from build123d import *

# Parameters (mm, degrees)
F0_W      = 139.7
F0_H      = 19.05
F1_DEPTH  = 6.35
F2_R      = 3.175
F3_DEPTH  = 6.351
F4_R      = 3.175
F5_DEPTH  = 25.4
F6_R      = 9.52499
F7_R      = 9.52499
F8_R      = 3.175
F9_DEPTH  = 6.351
F11_DEPTH = 6.35


# Not quite as in the source:
# - a fillet or chamfer is up to 0.001 mm smaller than in the source, because OpenCascade refuses the exact size


with BuildPart() as f1:
    # F0 (on Front) → F1 (new body)
    with BuildSketch(Plane.XZ):
        with Locations((69.85, 9.525)):
            Rectangle(F0_W, F0_H)
    extrude(amount=F1_DEPTH)

    # F2 (on face) → F3 (cut, through all)
    with BuildSketch(Plane.XZ.offset(6.35)):
        with Locations((130.175, 9.525)):
            Circle(F2_R)
    extrude(amount=-F3_DEPTH, mode=Mode.SUBTRACT)

    # F4 (on face) → F5 (cut)
    with BuildSketch(Plane.XZ.offset(6.35)):
        with Locations((104.775, 9.525)):
            Circle(F4_R)
    extrude(amount=-F5_DEPTH, mode=Mode.SUBTRACT)

    # F6 (radius 9.525 in the source; OpenCascade refuses exactly that, so slightly less here)
    f6_edges = [f1.edges().sort_by_distance(p)[0] for p in [
        (139.7, -3.175, 19.05),
        (139.7, -3.175, 0),
    ]]
    fillet(f6_edges, radius=F6_R)

    # F7 (radius 9.525 in the source; OpenCascade refuses exactly that, so slightly less here)
    f7_edges = [f1.edges().sort_by_distance(p)[0] for p in [
        (0, -3.175, 19.05),
        (0, -3.175, 0),
    ]]
    fillet(f7_edges, radius=F7_R)

    # F8 (on face) → F9 (cut, through all)
    with BuildSketch(Plane.XZ.offset(6.35)):
        with Locations((9.525, 9.525)):
            Circle(F8_R)
    extrude(amount=-F9_DEPTH, mode=Mode.SUBTRACT)

    # F10 (on face) → F11 (join)
    with BuildSketch(Plane.XZ.offset(6.35)):
        with BuildLine():
            Line((21.06826753, 38.1), (2.2284266793, 15.6475519823))
            ThreePointArc((2.2284266793, 15.6475519823), (5.4995610569, 18.1575816715), (9.525, 19.05))
            Line((9.525, 19.05), (81.5031155039, 19.05))
            Line((81.5031155039, 19.05), (65.51826753, 38.1))
            Line((65.51826753, 38.1), (21.06826753, 38.1))
        make_face()
    extrude(amount=-F11_DEPTH)


solid = f1.part
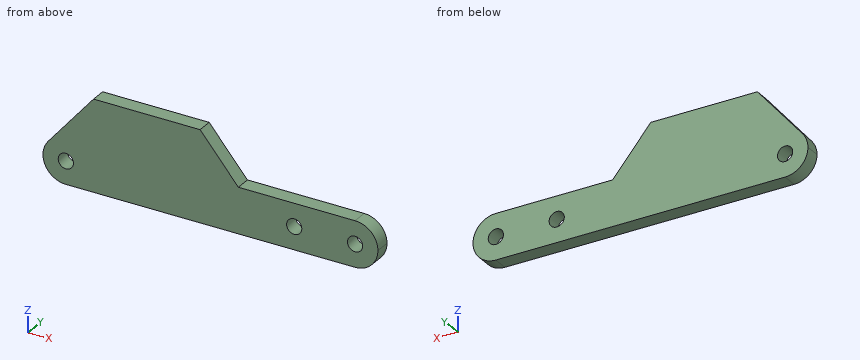
For this review, take the finished solid that the model builds, in its own axes (mm). Round coordinates to 2 decimals unless told otherwise and drop trailing zeros. Write each loop counter-clockwise with the first axis right and the second up, starting at its lowest first coordinate (ties: lowest second). Pieces come first, ordered by that corner, then holes. Notation, with made-up numbers: (-32, 68) - (-12, 68) arc R32 cw to (-12, 102) - close; hole circle Ø6 at (26, 77). An arc over 180 degrees is marked (long way). Write item = value, one per line. Start each with the question number.
1. Consider section C-C on z = 33. State the section outline as (x, y) points, plus the area to 3 significant figures.
2. For pin 1 Ø1 at (x, z) = (115, 21) entering from -Y; pin 2 Ø7.5 at (x, z) = (9.525, 9.525) entering from -Y; pin 3 Ø3 at (x, y) = (95.5, -4) entering from +Z, all flat-tipped, find the tip position at first contact; note any pin that passes through.
3. Consider section B-B on x = 119. State the section outline as (y, z) points.
4. Consider section A-A on y = -1. Give the number of separate pieces and of enclosed holes in the cut face, plus the area to 3 significant figures.
5. Wall thickness on L1, parallel to X at y = -3, z = 9; L2, parallel to Z at x = 111.5, y = -1.75; L3, parallel to Z at x = 8, y = -5.5: over which ranges is each line inside the solid? List them lowest first.
Evaluation:
q1.outline = (16.79, -6.35) - (69.8, -6.35) - (69.8, 0) - (16.79, 0) - close
q1.area = 337 mm2
q2.pin_1 = through
q2.pin_2 = -6.35
q2.pin_3 = 19.05
q3.outline = (-6.35, 0) - (0, 0) - (0, 19.05) - (-6.35, 19.05) - close
q4.separate_pieces = 1
q4.enclosed_holes = 3
q4.area = 3,640 mm2
q5.L1 = 0.01 to 6.39, 12.66 to 101.64, 107.91 to 127.04, 133.31 to 139.69
q5.L2 = 0 to 19.05
q5.L3 = 0.12 to 6.74, 12.31 to 22.53
